```python
from build123d import *

# Parameters (mm, degrees)
SKETCH2_W          = 628.65
SKETCH2_H          = 396.08125
EXTRUDE1_DEPTH     = 17.78
SKETCH3_R          = 15.08125
SKETCH3_R_2        = 3.4925
SKETCH3_R_3        = 1.5875
SKETCH3_W          = 308.0004
SKETCH3_H          = 261.9629
CUT_EXTRUDE1_DEPTH = 17.78
CUT_EXTRUDE2_DEPTH = 5.08
CUT_EXTRUDE4_DEPTH = 396.08125
FILLET1_R          = 20.6502


with BuildPart() as part:
    # Sketch2 → Extrude1 (new body)
    with BuildSketch(Plane.XY):
        with Locations((12009.966666666, -5854.303125)):
            Rectangle(SKETCH2_W, SKETCH2_H)
    extrude(amount=-EXTRUDE1_DEPTH)

    # Sketch3 → Cut-Extrude1 (cut)
    with BuildSketch(Plane.XY):
        with Locations((12267.141666666, -5761.0375)):
            Circle(SKETCH3_R)
        with Locations((12173.479166666, -5831.68125)):
            Circle(SKETCH3_R_2)
        with Locations((12266.824166666, -5865.01875)):
            Circle(SKETCH3_R_3)
        with Locations((12266.824166666, -5922.16875)):
            Circle(SKETCH3_R_3)
        with Locations((12266.824166666, -5979.31875)):
            Circle(SKETCH3_R_3)
        with Locations((12209.991666666, -6037.10375)):
            Circle(SKETCH3_R_3)
        with Locations((12009.966666666, -6037.10375)):
            Circle(SKETCH3_R_3)
        with Locations((11809.941666666, -6037.10375)):
            Circle(SKETCH3_R_3)
        with Locations((11753.109166666, -5979.31875)):
            Circle(SKETCH3_R_3)
        with Locations((11753.109166666, -5922.16875)):
            Circle(SKETCH3_R_3)
        with Locations((11753.109166666, -5865.01875)):
            Circle(SKETCH3_R_3)
        with Locations((11846.454166666, -5831.68125)):
            Circle(SKETCH3_R_2)
        with Locations((12009.966666666, -5972.175)):
            Circle(SKETCH3_R_2)
        with Locations((12009.966666666, -5691.1875)):
            Circle(SKETCH3_R_2)
        with Locations((12009.966666666, -5831.68125)):
            Rectangle(SKETCH3_W, SKETCH3_H)
        with BuildLine():
            Line((11734.654409808, -5693.754968556), (11739.23011943, -5693.754968556))
            ThreePointArc((11739.23011943, -5693.754968556), (11748.029166666, -5687.976468556), (11756.828213901, -5693.754968556))
            Line((11756.828213901, -5693.754968556), (11761.386355753, -5693.754968556))
            ThreePointArc((11761.386355753, -5693.754968556), (11767.531113043, -5692.357368906), (11771.079666666, -5697.564968556))
            ThreePointArc((11771.079666666, -5697.564968556), (11767.531113043, -5702.772568206), (11761.386355753, -5701.374968556))
            Line((11761.386355753, -5701.374968556), (11756.828213901, -5701.374968556))
            ThreePointArc((11756.828213901, -5701.374968556), (11754.760305425, -5704.393665595), (11751.712166666, -5706.417925308))
            Line((11751.712166666, -5706.417925308), (11751.712166666, -5721.30243896))
            ThreePointArc((11751.712166666, -5721.30243896), (11748.029166666, -5731.092968556), (11744.346166666, -5721.30243896))
            Line((11744.346166666, -5721.30243896), (11744.346166666, -5706.417925308))
            ThreePointArc((11744.346166666, -5706.417925308), (11741.298027907, -5704.393665595), (11739.23011943, -5701.374968556))
            Line((11739.23011943, -5701.374968556), (11734.654409809, -5701.374968556))
            ThreePointArc((11734.654409809, -5701.374968556), (11724.978666666, -5697.564968556), (11734.654409808, -5693.754968556))
        make_face()
    extrude(amount=-CUT_EXTRUDE1_DEPTH, mode=Mode.SUBTRACT)

    # Sketch4 → Cut-Extrude2 (cut)
    with BuildSketch(Plane.XY):
        Polygon((11975.041666666, -6028.21375), (11695.641666666, -6028.21375), (11695.641666666, -6045.99375), (12324.291666666, -6045.99375), (12324.291666666, -6028.21375), align=None)
    extrude(amount=-CUT_EXTRUDE2_DEPTH, mode=Mode.SUBTRACT)

    # Sketch7 → Cut-Extrude4 (cut)
    with BuildSketch(Plane.XZ.offset(6052.34375)):
        Polygon((11701.991666666, -11.43), (11701.991666666, 0), (11695.641666666, 0), (11695.641666666, -17.78), align=None)
        Polygon((12317.941666666, -11.43), (12324.291666666, -17.78), (12324.291666666, 0), (12317.941666666, 0), align=None)
    extrude(amount=-CUT_EXTRUDE4_DEPTH, mode=Mode.SUBTRACT)

    # Fillet1
    fillet1_edges = [part.edges().sort_by_distance(p)[0] for p in [
        (11855.966466666, -5962.6627, -8.89),
        (11855.966466666, -5700.6998, -8.89),
        (12163.966866666, -5700.6998, -8.89),
        (12163.966866666, -5962.6627, -8.89),
    ]]
    fillet(fillet1_edges, radius=FILLET1_R)


solid = part.part
```
Model file for the job. Use its own axes, mm. A direction names the side the tool comes from. Round coordinates to 2 decimals unless told otherwise and drop trailing zeros. Write each loop counter-clockwise with the first axis right and the second up, starting at its lowest first coordinate (ties: lowest second). Pieces come first, ordered by that corner, then holes. Notation, with made-up numbers: (-24, -9) - (21, -9) arc R21 ccw to (21, 2) - close; hole circle Ø4 at (66, 43). An arc over 180 degrees is marked (long way). Use CSV: the item, a comma, the result in double quotes. Start each with the question number.
Item 1: Band-saw the part on B-B (y = -5844). Write the cut outline in (x, z), and give its area (3 significant figures).
Item 2: Pin check, flat tips, straight feed: P1, Ø5.5, axis at x = 11919.5, y = -6036.5, coming from the +Z side; P2, Ø4, axis at y = -5975.5, z = -12.5, coming from the +X side; P3, Ø5.5, axis at y = -5865.5, z = -7.5, coming from the -X side. Stop position of each tip, or through.
Item 3: Drill centre lines: L1, parallel to Y at x = 11928, z = -2.5; L2, parallel to Y at x = 12142, z = -15.5; L3, parallel to X at y = -5706, z = -13. Where is each one in solid material? Low to high. Write a range as [from, to].
Item 4: Band-saw the part on A-A (x = 12114.5). Write the cut outline in (y, z).
Item 5: Tool access for faces 4 (the face through (12008, -5962.663, -9)), 5 (the face through (12006, -5964, 0)), 6 (the face through (12006, -6037, -5.08)): list every direction of +Z, -Z, +X, -X, +Y, -Y with a clear straight run to the whole face (end or side of a thin tool).
Item 6: Two-plate mould, pull along X, no slides. Class faces 1 (the face through (12006, -5984, -17.78)), 2 (the face through (11701.992, -5857, -6)), 3 (the face through (12157.76, -5956.77, -9.01)): released by +X, released by -X, zero draft, split by the parting line, or undercut.
Item 7: Band-saw the part on C-C (z = -8.5). State how many separate pieces and enclosed holes the cut face has, and give its area (3 significant figures).
Checked values:
1,outline,"(11695.64, -17.78) - (11855.97, -17.78) - (11855.97, 0) - (11701.99, 0) - (11701.99, -11.43) - close; (12163.97, -17.78) - (12324.29, -17.78) - (12317.94, -11.43) - (12317.94, 0) - (12163.97, 0) - close"
1,area,"5,520 mm²"
2,P1,"stops at z = -5.08"
2,P2,"stops at x = 12321.01"
2,P3,"stops at x = 11701.99"
3,L1,"y = [-6052.34, -6045.99], [-6028.21, -5962.66], [-5700.7, -5656.26]"
3,L2,"y = [-6052.34, -5962.66], [-5700.7, -5656.26]"
3,L3,"x = [11700.42, 11743.47], [11752.59, 11862.8], [12157.13, 12319.51]"
4,outline,"(-6052.34, -17.78) - (-5962.66, -17.78) - (-5962.66, 0) - (-6028.21, 0) - (-6028.21, -5.08) - (-6045.99, -5.08) - (-6045.99, 0) - (-6052.34, 0) - close; (-5700.7, -17.78) - (-5656.26, -17.78) - (-5656.26, 0) - (-5700.7, 0) - close"
5,face 4,"+Z, -Z"
5,face 5,"+Z, +X, -X, +Y, -Y"
5,face 6,"+Z, +X, -X"
6,face 1,"zero draft"
6,face 2,"released by -X"
6,face 3,"undercut"
7,separate pieces,"1"
7,enclosed holes,"16"
7,area,"162,000 mm²"
